from build123d import *

# Parameters (mm, degrees)
F1_DEPTH = 0.381
F2_R     = 3.175
F3_DEPTH = 7.62
F4_R     = 1.5875
F5_DEPTH = 7.62


with BuildPart() as f1:
    # F0 (on Front) → F1 (new body, symmetric)
    with BuildSketch(Plane.XZ):
        with BuildLine():
            Line((0, 22.5393476782), (0, 0))
            ThreePointArc((0, 0), (5.7666386867, 3.691357817), (4.8287964934, 10.4737391315))
            ThreePointArc((4.8287964934, 10.4737391315), (3.0115337416, 15.7752394789), (5.3116761428, 20.8857868838))
            ThreePointArc((5.3116761428, 20.8857868838), (7.399265484, 24.5285593059), (7.2405055752, 28.7241064059))
            Line((7.2405055752, 28.7241064059), (0, 50.8))
            Line((0, 50.8), (0, 30.1593476782))
            ThreePointArc((0, 30.1593476782), (2.6940768363, 29.0434245145), (3.81, 26.3493476782))
            ThreePointArc((3.81, 26.3493476782), (2.6940768363, 23.6552708418), (0, 22.5393476782))
        make_face()
        with BuildLine():
            ThreePointArc((-4.8287964934, 10.4737391315), (-5.7666386867, 3.691357817), (0, 0))
            Line((0, 0), (0, 22.5393476782))
            ThreePointArc((0, 22.5393476782), (-3.81, 26.3493476782), (0, 30.1593476782))
            Line((0, 30.1593476782), (0, 50.8))
            Line((0, 50.8), (-7.2405055752, 28.7241064059))
            ThreePointArc((-7.2405055752, 28.7241064059), (-7.399265484, 24.5285593059), (-5.3116761428, 20.8857868838))
            ThreePointArc((-5.3116761428, 20.8857868838), (-3.0115337416, 15.7752394789), (-4.8287964934, 10.4737391315))
        make_face()
    extrude(amount=F1_DEPTH, both=True)

    # F2 (on face) → F3 (join)
    with BuildSketch(Plane(origin=(0, 0.381, 0), x_dir=(-1, 0, 0), z_dir=(0, 1, 0))):
        with Locations((0, 6.35)):
            Circle(F2_R)
    extrude(amount=F3_DEPTH)

    # F4 (on face) → F5 (cut)
    with BuildSketch(Plane(origin=(0, 8.001, 0), x_dir=(-1, 0, 0), z_dir=(0, 1, 0))):
        with Locations((0, 6.35)):
            Circle(F4_R)
    extrude(amount=-F5_DEPTH, mode=Mode.SUBTRACT)


solid = f1.part
Check sheet for the modelled part. Datum: model origin and axes. Units: mm. A direction names the side the tool comes from. Coordinates: 2 decimals unless noted, no trailing zeros. Loops run counter-clockwise (first coordinate to the right, second up) from the corner with the lowest first, then second, coordinate; pieces in that order, holes last. Notation, with made-up numbers: (58, 43) -> (112, 43) arc R17 cw to (112, 59) -> close; hole circle Ø2 at (67, 33.25). An arc over 180 degrees is marked (long way). Write item = value, one per line. Start each with the question number.
1. Section check A-A on x = -0.5. Record the cut outline in (y, z).
2. Tool access check on faces 4 (the flat face through (0, -0.381, 20)), 5 (the flat face through (0, 0.381, 6)). Record the directions out of +Z, -Z, +X, -X, +Y, -Y that give a thin tool (end or side, any length) a straight path to the whole face; none if there is none.
3. Material ranges on line 1 (Z direction, x = 0, y = 3.5) (1 decimal); line 2 (Y direction, x = -0.5, z = 17.5); line 3 (X direction, y = 0.25, z = 23.5), recorded low to high.
4. Depth check by flat-ended pin: P1, Ø6, axis at x = 4, z = 31.5, coming from the +Y side; P2, Ø5, axis at x = 1.5, y = 7, coming from the +Z side (3 decimals). Enter the tip coordinate at first touch or a pass-through.
5. Draft check along X on faces 1 (the flat face through (-1, 8.001, 8)), 2 (the cylindrical face through (-0.73, 4.24, 4.94)), 3 (the cylindrical face through (-1.707, 4.138, 9.027)). Enter one of: released by +X, released by -X, zero draft, split by the parting line, or undercut.
6. Section check B-B on z = 23.5. Record the cut outline in (x, y).
Responses:
q1.outline = (-0.38, 0.02) -> (0.38, 0.02) -> (0.38, 3.21) -> (8, 3.21) -> (8, 4.84) -> (0.38, 4.84) -> (0.38, 7.86) -> (8, 7.86) -> (8, 9.49) -> (0.38, 9.49) -> (0.38, 22.57) -> (-0.38, 22.57) -> close; (-0.38, 30.13) -> (0.38, 30.13) -> (0.38, 49.28) -> (-0.38, 49.28) -> close
q2.face_4 = +Z, -Z, +X, -X, -Y
q2.face_5 = +Y
q3.line_1 = 3.2 to 4.8, 7.9 to 9.5
q3.line_2 = -0.38 to 0.38
q3.line_3 = -7.07 to -2.53, 2.53 to 7.07
q4.P1 = 0.38
q4.P2 = 9.525
q5.face_1 = zero draft
q5.face_2 = undercut
q5.face_3 = split by the parting line
q6.outline = (-7.07, -0.38) -> (-2.53, -0.38) -> (-2.53, 0.38) -> (-7.07, 0.38) -> close; (2.53, -0.38) -> (7.07, -0.38) -> (7.07, 0.38) -> (2.53, 0.38) -> close
